Here's how the part is built. I have some questions about the finished solid (model axes, mm). Face numbers are marked on the shaded views. Round coordinates to 2 decimals unless told otherwise and drop trailing zeros. Loops run counter-clockwise (first coordinate to the right, second up) from the corner with the lowest first, then second, coordinate; pieces in that order, holes last. Notation, with made-up numbers: (-25, 4) - (20, 4) arc R20 cw to (20, 24) - close; hole circle Ø7 at (25.5, -34). An arc over 180 degrees is marked (long way). Answer as a JSON object with one key per item and string values. Group by question number.
1) Will this pin go through, and if not, where does the flat tip stop? P1, Ø3, axis at x = -3.5, y = -0.5, coming from the -Z side.
2) I want a section at A-A, the plane x = -7. Please give me the cut outline in (y, z), then the cut area to 3 significant figures.
3) I want a section at C-C, the plane z = 1.05. Give the number of separate pieces and of enclosed holes in the cut face, then the cut area to 3 significant figures.
4) If we mould it in two halves opening along X, with no side actions, what happens to the marked faces 1, 2, 3 and 4? For each: pulls with the +X half, pulls with the -X half, needs draft (parallel to the pull), parting line crosses it, or undercut.
5) I want a section at B-B, the plane y = 0. Please give me the cut outline in (x, z).
6) I want a section at D-D, the plane x = 5. Please give me the cut outline in (y, z).
7) If I drill on line 1 along Y through (x, z) = (5, 1.45); line 2 along X through (y, z) = (-1.25, 0.2); line 3 along X through (y, z) = (-1, 2.1), over which ranges is the centre line in solid material (lowest first)? Write a range as [from, to].
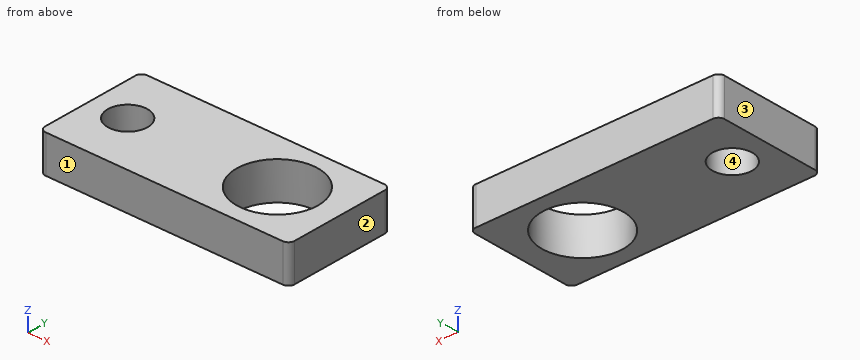
Solid Edge part; units mm, degrees
sketch "Sketch1" plane through (0, 0, 0) normal (0, 0, 1) x (1, 0, 0)
  line L0 (10, -4.5) -> (-10, -4.5)
  line L1 (-10, -4.5) -> (-10, 4.5)
  line L2 (-10, 4.5) -> (10, 4.5)
  line L3 (10, 4.5) -> (10, -4.5)
  circle A0 centre (5, 0) radius 3.25
  circle A1 centre (-7, 0) radius 1.5875
extrude "Protrusion1" add sketch "Sketch1" along normal blind 3
fillet "Round_1" radius 0.5 4 edges at (10, -4.5, 1.5) (10, 4.5, 1.5) (-10, 4.5, 1.5) (-10, -4.5, 1.5)
Outcome:
{
 "1": {"P1": "z = 0"},
 "2": {"outline": "(-4.5, 0) - (-1.59, 0) - (-1.59, 3) - (-4.5, 3) - close; (1.59, 0) - (4.5, 0) - (4.5, 3) - (1.59, 3) - close", "area": "17.5 mm^2"},
 "3": {"separate pieces": "1", "enclosed holes": "2", "area": "139 mm^2"},
 "4": {"face 1": "needs draft", "face 2": "pulls with the +X half", "face 3": "pulls with the -X half", "face 4": "undercut"},
 "5": {"outline": "(-10, 0) - (-8.59, 0) - (-8.59, 3) - (-10, 3) - close; (-5.41, 0) - (1.75, 0) - (1.75, 3) - (-5.41, 3) - close; (8.25, 0) - (10, 0) - (10, 3) - (8.25, 3) - close"},
 "6": {"outline": "(-4.5, 0) - (-3.25, 0) - (-3.25, 3) - (-4.5, 3) - close; (3.25, 0) - (4.5, 0) - (4.5, 3) - (3.25, 3) - close"},
 "7": {"line 1": "[-4.5, -3.25], [3.25, 4.5]", "line 2": "[-10, -7.98], [-6.02, 2], [8, 10]", "line 3": "[-10, -8.23], [-5.77, 1.91], [8.09, 10]"}
}
